Read the model definition and answer for the solid it produces. Units are mm, in the model's axes. A direction names the side the tool comes from. Give positions to 0.01 mm unless a question says otherwise; leave off trailing zeros. Write each loop counter-clockwise with the first axis right and the second up, starting at its lowest first coordinate (ties: lowest second). Pieces come first, ordered by that corner, then holes. Notation, with made-up numbers: M 22.5,-38 L 41.5,-38 A21 cw 41.5,-22 Z; hole C 26.5,-3.75 d8. An arc over 180 degrees is marked long. Put each result on its own line as item: value.
from build123d import *

# Parameters (mm, degrees)
SKETCH1_R           = 80
BOSS_EXTRUDE1_DEPTH = 200
SKETCH2_R           = 44
BOSS_EXTRUDE2_DEPTH = 14
SKETCH3_R           = 30
BOSS_EXTRUDE3_DEPTH = 7
SKETCH4_R           = 21.5
CUT_EXTRUDE1_DEPTH  = 7


with BuildPart() as part:
    # Sketch1 → Boss-Extrude1 (new body)
    with BuildSketch(Plane.XY):
        Circle(SKETCH1_R)
    extrude(amount=BOSS_EXTRUDE1_DEPTH)

    # Sketch2 → Boss-Extrude2 (add)
    with BuildSketch(Plane(origin=(0, 0, 0), x_dir=(-1, 0, 0), z_dir=(0, 0, -1))):
        Circle(SKETCH2_R)
    extrude(amount=BOSS_EXTRUDE2_DEPTH)

    # Sketch3 → Boss-Extrude3 (add)
    with BuildSketch(Plane(origin=(0, 0, -14), x_dir=(-1, 0, 0), z_dir=(0, 0, -1))):
        Circle(SKETCH3_R)
    extrude(amount=BOSS_EXTRUDE3_DEPTH)

    # Sketch4 → Cut-Extrude1 (cut)
    with BuildSketch(Plane(origin=(0, 0, -21), x_dir=(-1, 0, 0), z_dir=(0, 0, -1))):
        Circle(SKETCH4_R)
    extrude(amount=-CUT_EXTRUDE1_DEPTH, mode=Mode.SUBTRACT)


solid = part.part
(1) Section D-D on x = 39 is taken. Determine the outline of the cut face in (y, z).
Result:
outline: M -69.85,0 L -20.37,0 L -20.37,-14 L 20.37,-14 L 20.37,0 L 69.85,0 L 69.85,200 L -69.85,200 Z
(2) Section C-C on z = 30 is taken. Determine the outline of the cut face in (x, y), and give its area (3 significant figures).
Result:
outline: C 0,0 d160
area: 20,100 mm²
(3) For a pull along Y with two mould halves and no side action, classify faces 1 (the face through (2.799, 21.317, -17.549)), 2 (the face through (-17.34, -78.1, 98.6)), 3 (the face through (-29, -9, -14)) as +Y half, -Y half, draft (parallel to the pull), parting line (faces both ways), or undercut.
Result:
face 1: undercut
face 2: parting line
face 3: draft
(4) Straight lines are drawn through the part: line 1 along Y through (x, z) = (0, -16); line 2 along Z through (x, y) = (-6.5, 56); line 3 along Y through (x, z) = (3, 27). For each, find the intervals that lie inside material, in ascending order. Write a range as from..to.
Result:
line 1: y = -30..-21.5, 21.5..30
line 2: z = 0..200
line 3: y = -79.94..79.94
(5) Given pin 1 Ø10 at (y, z) = (-17, 164.5) entering from -X; pin 2 Ø1.5 at (y, z) = (-23, 152.5) entering from +X; pin 3 Ø1.5 at (x, z) = (-29.5, 79) entering from -Y, each flat-ended and moving along its own axis, determine where each tip first touches the part or whether it passes through.
Result:
pin 1: stops at x = -79.09
pin 2: stops at x = 76.84
pin 3: stops at y = -74.66
(6) Which of the six approach directions +Z, -Z, +X, -X, +Y, -Y give full straight-line access (tool end or side, diameter ignored) to faces 4 (the face through (9.538, -42.954, -6.902)), 5 (the face through (-1, 1, 200))?
Result:
face 4: -Z
face 5: +Z, +X, -X, +Y, -Y
(7) Section A-A on y = 0 is taken. Determine the outline of the cut face in (x, z).
Result:
outline: M -80,0 L -44,0 L -44,-14 L -30,-14 L -30,-21 L -21.5,-21 L -21.5,-14 L 21.5,-14 L 21.5,-21 L 30,-21 L 30,-14 L 44,-14 L 44,0 L 80,0 L 80,200 L -80,200 Z
